Part print with two shaded views. Sizes in mm from the minimum x, y, z corner. Round coordinates to 2 decimals unless told otherwise and drop trailing zeros. Loops run counter-clockwise (first coordinate to the right, second up) from the corner with the lowest first, then second, coordinate; pieces in that order, holes last. Notation, with made-up numbers: (73, 71) -> (128, 71) arc R25 cw to (128, 101) -> close; hole circle Ø11 at (2, 50.5). An arc over 180 degrees is marked (long way). Use a Markdown table: item, result. Add a question column.
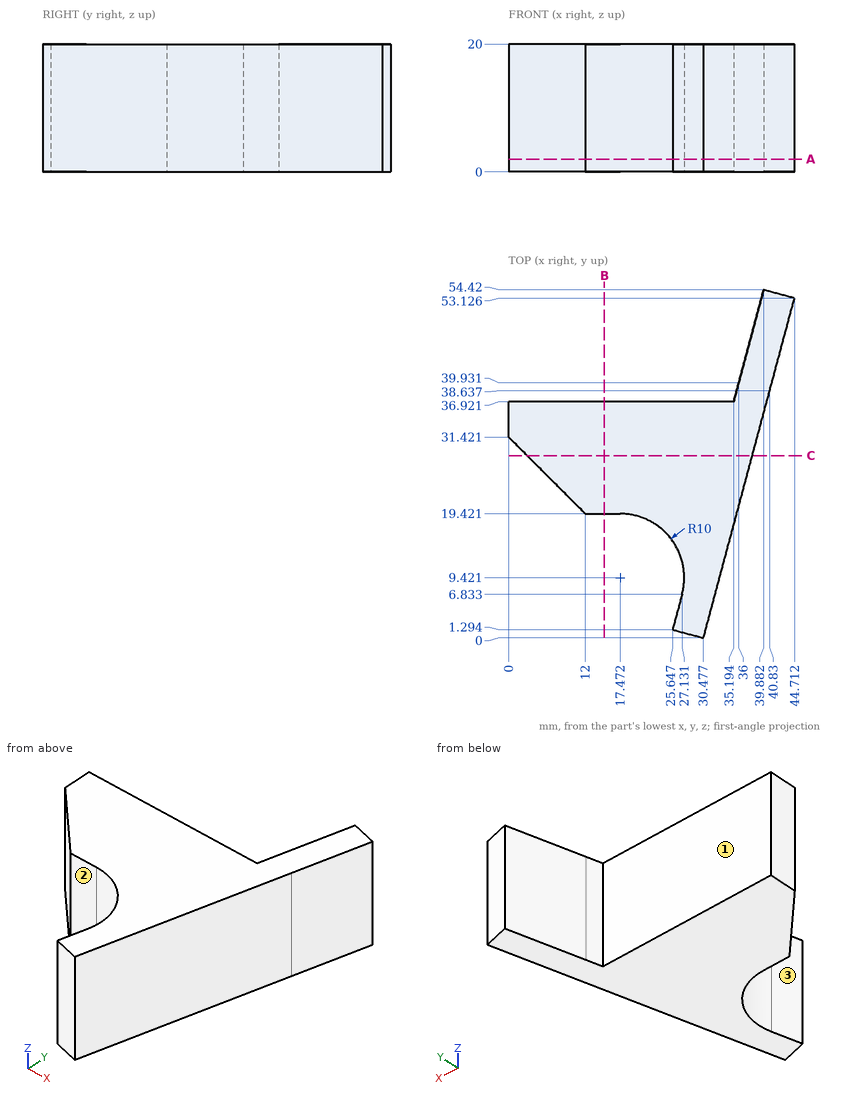
1) Pin check, flat tips, straight feed: pin 1 Ø10 at (x, z) = (23.5, 15.5) entering from -Y; pin 2 Ø4 at (y, z) = (9.5, 11.5) entering from -X; pin 3 Ø6 at (x, z) = (30.5, 12) entering from +Y. Stop position of each tip, or through.
2) Cut at B-B on x = 15. Write the cut outline in (y, z), and give its area (3 significant figures).
3) Wall check: probe 1 along Y at (x, z) = (18, 14); probe 2 along Y at (x, z) = (6, 9.25); probe 3 along X at (y, z) = (8.5, 8.5) (1 decimal). Give the ranges that are in metal, low to high. Write a range as from..to.
4) Pull direction Y, two halves, no side cores. Call the marked faces 1, 2 and 3: +Y half, -Y half, draft (parallel to the pull), parting line (faces both ways), or undercut.
5) Cut at A-A on z = 2. Write the cut outline in (x, y) (1 decimal).
6) Cut at C-C on y = 28.5. Write the cut outline in (x, z), and give its area (3 significant figures).
Established:
| question | item | result |
|---|---|---|
| 1 | pin 1 | stops at y = 0.53 |
| 1 | pin 2 | stops at x = 27.25 |
| 1 | pin 3 | stops at y = 36.92 |
| 2 | outline | (19.42, 0) -> (36.92, 0) -> (36.92, 20) -> (19.42, 20) -> close |
| 2 | area | 350 mm^2 |
| 3 | probe 1 | y = 19.41..36.92 |
| 3 | probe 2 | y = 25.42..36.92 |
| 3 | probe 3 | x = 27.4..32.8 |
| 4 | face 1 | +Y half |
| 4 | face 2 | -Y half |
| 4 | face 3 | undercut |
| 5 | outline | (0, 31.4) -> (12, 19.4) -> (17.5, 19.4) arc R10 cw to (27.1, 6.8) -> (25.6, 1.3) -> (30.5, 0) -> (40.8, 38.6) -> (44.7, 53.1) -> (39.9, 54.4) -> (36, 39.9) -> (35.2, 36.9) -> (0, 36.9) -> close |
| 6 | outline | (2.92, 0) -> (38.11, 0) -> (38.11, 20) -> (2.92, 20) -> close |
| 6 | area | 704 mm^2 |
